Autodesk Fusion 360 part; units mm, degrees
sketch "スケッチ1" plane through (0, 0, 0) normal (0, 0, 1) x (1, 0, 0)
  line L0 (0, 0) -> (84, 0)
  line L1 (84, 0) -> (84, 40)
  line L2 (84, 40) -> (0, 40)
  line L3 (0, 40) -> (0, 0)
  dimension "d1" = 40
  dimension "d2" = 84
extrude "押し出し1" add sketch "スケッチ1" along normal blind 32
sketch "スケッチ2" plane through (0, 0, 32) normal (0, 0, 1) x (-1, 0, 0)
  line L0 (0, -40) -> (0, 0)
  line L1 (0, 0) -> (-84, 0)
  line L2 (-84, 0) -> (-84, -40)
  line L3 (-84, -40) -> (0, -40)
  line L4 (-9, -32.5) -> (-51, -32.5)
  line L5 (-51, -32.5) -> (-51, -7.5)
  line L6 (-51, -7.5) -> (-9, -7.5)
  line L7 (-9, -7.5) -> (-9, -32.5)
  dimension "d5" = 42
  dimension "d6" = 25
  dimension "d27" = 9
  dimension "d72" = 7.5
extrude "押し出し2" cut sketch "スケッチ2" against normal blind 20 contours L4 L5 L6 L7
fillet "フィレット1" radius 1 4 edges at (84, 0, 16) (84, 40, 16) (0, 0, 16) (0, 40, 16)
sketch "スケッチ5" plane through (0, 0, 32) normal (0, 0, 1) x (-1, 0, 0)
  arc A0 (-1, -40) -> (0, -39) centre (-1, -39) ccw
  line L0 (0, -39) -> (0, -1)
  arc A1 (0, -1) -> (-1, 0) centre (-1, -1) ccw
  line L1 (-1, 0) -> (-83, 0)
  arc A2 (-83, 0) -> (-84, -1) centre (-83, -1) ccw
  line L2 (-84, -1) -> (-84, -39)
  arc A3 (-84, -39) -> (-83, -40) centre (-83, -39) ccw
  line L3 (-83, -40) -> (-1, -40)
  line L4 (-51, -32.5) -> (-51, -7.5)
  line L5 (-51, -7.5) -> (-9, -7.5)
  line L6 (-9, -7.5) -> (-9, -32.5)
  line L7 (-9, -32.5) -> (-51, -32.5)
  circle A4 centre (-5, -5) radius 2.5
  circle A5 centre (-5, -35) radius 2.5
  circle A6 centre (-79, -5) radius 2.5
  circle A7 centre (-79, -35) radius 2.5
  dimension "d28" = 5
  dimension "d29" = 5
  dimension "d30" = 5
  dimension "d31" = 5
  dimension "d32" = 5
  dimension "d33" = 5
  dimension "d34" = 5
  dimension "d35" = 5
  dimension "d36" = 5
  dimension "d37" = 5
  dimension "d38" = 5
  dimension "d39" = 5
extrude "押し出し4" cut sketch "スケッチ5" against normal blind 8 contours A4 | A5 | A6 | A7
sketch "スケッチ18" plane through (0, 0, 0) normal (0, -1, 0) x (1, 0, 0)
  line L0 (1, 32) -> (1, 0)
  line L1 (1, 0) -> (83, 0)
  line L2 (83, 0) -> (83, 32)
  line L3 (83, 32) -> (1, 32)
  line L4 (1, 1) -> (83, 1)
  line L5 (83, 1) -> (83, 10)
  line L6 (83, 10) -> (1, 10)
  line L7 (1, 10) -> (1, 1)
  dimension "d75" = 9
extrude "押し出し16" cut sketch "スケッチ18" against normal blind 40 contours L0 L2 L4 L5 L6 L7
Read the model definition and answer for the solid it produces. Units are mm, in the model's axes. A direction names the side the tool comes from. Give positions to 0.01 mm unless a question says otherwise; leave off trailing zeros. Order: outer loops, then holes, each group sorted by start corner. A loop starts at its lowest first (then second) coordinate and runs counter-clockwise, first axis right, second up. Notation, with made-up numbers: (48, 74) -> (98, 74) arc R14 cw to (98, 101) -> close; hole circle Ø9 at (58.25, -12.5). An arc over 180 degrees is marked (long way). Write item = value, one per line.
1. A cutting plane is placed at D-D, the plane z = 8.5. Write down the section's boundary in (x, y).
Numbers:
outline = (0, 1) arc R1 ccw to (1, 0) -> (1, 40) arc R1 ccw to (0, 39) -> close; (83, 0) arc R1 ccw to (84, 1) -> (84, 39) arc R1 ccw to (83, 40) -> close
2. A cutting plane is placed at A-A, the plane y = 30.5. Write down the section's boundary in (x, z), and give its area (3 significant figures).
Numbers:
outline = (0, 0) -> (84, 0) -> (84, 32) -> (51, 32) -> (51, 12) -> (9, 12) -> (9, 32) -> (0, 32) -> close; hole (1, 1) -> (83, 1) -> (83, 10) -> (1, 10) -> close
area = 1,110 mm²
3. Straight lines are drawn through the part: line 1 along X through (y, z) = (35, 28); line 2 along Y through (x, z) = (5, 28); line 3 along Z through (x, y) = (74, 8). For each, find the intervals that lie inside material, in ascending order.
Numbers:
line_1 = 0 to 2.5, 7.5 to 76.5, 81.5 to 84
line_2 = 0 to 2.5, 7.5 to 32.5, 37.5 to 40
line_3 = 0 to 1, 10 to 32
4. A cutting plane is placed at C-C, the plane z = 30.5. Write down the section's boundary in (x, y), and give its area (3 significant figures).
Numbers:
outline = (0, 1) arc R1 ccw to (1, 0) -> (83, 0) arc R1 ccw to (84, 1) -> (84, 39) arc R1 ccw to (83, 40) -> (1, 40) arc R1 ccw to (0, 39) -> close; hole circle Ø5 at (5, 5); hole circle Ø5 at (5, 35); hole (9, 7.5) -> (51, 7.5) -> (51, 32.5) -> (9, 32.5) -> close; hole circle Ø5 at (79, 5); hole circle Ø5 at (79, 35)
area = 2,230 mm²
5. A cutting plane is placed at B-B, the plane x = 52. Write down the section's boundary in (y, z), and give its area (3 significant figures).
Numbers:
outline = (0, 0) -> (40, 0) -> (40, 1) -> (0, 1) -> close; (0, 10) -> (40, 10) -> (40, 32) -> (0, 32) -> close
area = 920 mm²
6. Given pin 1 (2.5 mm diameter, centred on x = 79, y = 36, fed in from +Z); pin 2 (1.5 mm diameter, centred on x = 72, z = 24, fed in from -Y), each flat-ended and moving along its own axis, determine where each tip first touches the part or whether it passes through.
Numbers:
pin_1 = 24
pin_2 = 0
7. For faces 4 (the face through (43, 40, 21)), 5 (the face through (30, 32.5, 22)), 6 (the face through (83, 20, 5)), determine the directions among +Z, -Z, +X, -X, +Y, -Y from which every point of the face is accessible in a straight line to the end or side of a thin tool.
Numbers:
face_4 = +Z, -Z, +X, -X, +Y
face_5 = +Z
face_6 = +Y, -Y
8. The mould has two halves that part along X. Classify faces 1 (the face through (51, 20, 22)), 2 (the face through (41, 20, 0)), 3 (the face through (84, 20, 16)): +X half, -X half, draft (parallel to the pull), parting line (faces both ways), or undercut.
Numbers:
face_1 = undercut
face_2 = draft
face_3 = +X half
